Drawing for the job (mm, zero at the part's lowest x, y, z). A direction names the side the tool comes from. Round coordinates to 2 decimals unless told otherwise and drop trailing zeros. Order: outer loops, then holes, each group sorted by start corner. A loop starts at its lowest first (then second) coordinate and runs counter-clockwise, first axis right, second up. Notation, with made-up numbers: (80, -34.5) - (134, -34.5) arc R19 ccw to (134, -12.5) - close; hole circle Ø11 at (64, 61.25). An arc over 180 degrees is marked (long way). Put each result on its own line as item: value. Start each with the question number.
Item 1: Saw through at C-C on x = 33.5. List the corners of the cut face in (y, z), plus the area to 3 significant figures.
Item 2: Saw through at B-B on y = 6. State how many separate pieces and enclosed holes the cut face has, plus the area to 3 significant figures.
Item 3: Saw through at A-A on z = 12.7. List the corners of the cut face in (x, y).
Item 4: Pin check, flat tips, straight feed: pin 1 Ø2.5 at (y, z) = (27.686, 12.7) entering from +X; pin 2 Ø1.5 at (x, y) = (31.5, 28.5) entering from -Z; pin 3 Ø8 at (x, z) = (37, 14) entering from +Y. Stop position of each tip, or through.
Item 5: Which spindle directions (+Z, -Z, +X, -X, +Y, -Y) get a long thin tool onto all of the face, cutting with end or side? Do the marked faces 1 and 2. Say none if no direction does.
Item 6: Mould opens along X. For the marked faces 3, 4 and 5 say: pulls with the +X half, pulls with the -X half, needs draft (parallel to the pull), parting line crosses it, or undercut.
Item 7: Saw through at D-D on x = 22. List the corners of the cut face in (y, z) (1 decimal), plus the area to 3 significant figures.
Item 8: Probe probe 1 along Y at (x, z) = (39.5, 12.7); probe 2 along Y at (x, z) = (38.5, 11.5) (1 decimal); probe 3 along Y at (x, z) = (32.5, 28). List the from-to ranges inside material, lowest first.
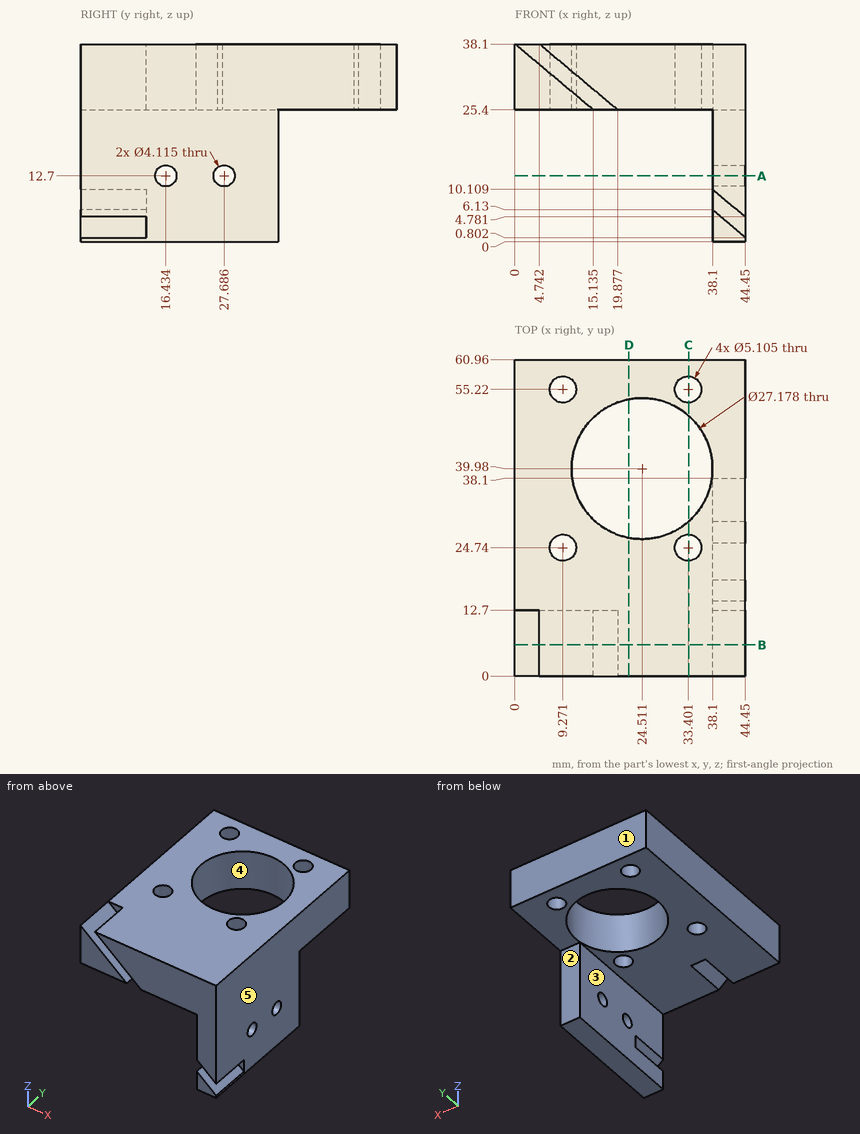
Results found:
1. outline: (0, 25.4) - (22.19, 25.4) - (22.19, 38.1) - (0, 38.1) - close; (27.29, 25.4) - (29.79, 25.4) - (29.79, 38.1) - (27.29, 38.1) - close; (50.17, 25.4) - (52.67, 25.4) - (52.67, 38.1) - (50.17, 38.1) - close; (57.77, 25.4) - (60.96, 25.4) - (60.96, 38.1) - (57.77, 38.1) - close
1. area: 386 mm²
2. separate pieces: 3
2. enclosed holes: 0
2. area: 640 mm²
3. outline: (38.1, 0) - (44.45, 0) - (44.45, 14.38) - (38.1, 14.38) - close; (38.1, 18.49) - (44.45, 18.49) - (44.45, 25.63) - (38.1, 25.63) - close; (38.1, 29.74) - (44.45, 29.74) - (44.45, 38.1) - (38.1, 38.1) - close
4. pin 1: passes through
4. pin 2: stops at z = 25.4
4. pin 3: stops at y = 38.1
5. face 1: +Z, -Z, +X, -X, +Y
5. face 2: -Z, +X, -X, +Y
6. face 3: pulls with the -X half
6. face 4: undercut
6. face 5: pulls with the +X half
7. outline: (0, 25.4) - (26.6, 25.4) - (26.6, 38.1) - (0, 38.1) - close; (53.3, 25.4) - (61, 25.4) - (61, 38.1) - (53.3, 38.1) - close
7. area: 435 mm²
8. probe 1: y = 0 to 14.38, 18.49 to 25.63, 29.74 to 38.1
8. probe 2: y = 0 to 14.8, 18.1 to 26, 29.4 to 38.1
8. probe 3: y = 0 to 22.35, 27.13 to 28.99, 50.97 to 52.83, 57.61 to 60.96
